For this review, take the finished solid that the model builds, in its own axes (mm). Face numbers are marked on the shaded views. Round coordinates to 2 decimals unless told otherwise and drop trailing zeros. Loops run counter-clockwise (first coordinate to the right, second up) from the corner with the lowest first, then second, coordinate; pieces in that order, holes last.
```python
from build123d import *

# Parameters (mm, degrees)
FILLET_4_R = 0.2
FILLET_5_R = 1


with BuildPart() as part:
    # Эскиз1 → Повернуть1 (revolve)
    with BuildSketch(Plane.XY, mode=Mode.PRIVATE) as revolve_1_sk:
        Polygon((-22.392450879, 1.834990157), (-22.392450879, 2.25), (-10.392450879, 2.25), (-9.392450879, 1.5), (-2.392450879, 1.5), (2.607549121, 1.05), (2.607549121, 0.75), (-2.663312046, 1.1), (-9.392450879, 1.1), (-10.602717789, 1.834990157), align=None)
    revolve(revolve_1_sk.sketch.rotate(Axis((-52.441675284, 0, 0), (1, 0, 0)), 90), axis=Axis((-52.441675284, 0, 0), (1, 0, 0)))

    # Скругление4
    fillet_4_edges = [part.edges().sort_by_distance(p)[0] for p in [
        (-22.392450879, 0, -2.25),
        (2.607549121, 0, -1.05),
    ]]
    fillet(fillet_4_edges, radius=FILLET_4_R)

    # Скругление5
    fillet_5_edges = [part.edges().sort_by_distance(p)[0] for p in [
        (-10.392450879, 0, -2.25),
        (-9.392450879, 0, -1.5),
    ]]
    fillet(fillet_5_edges, radius=FILLET_5_R)


solid = part.part
```
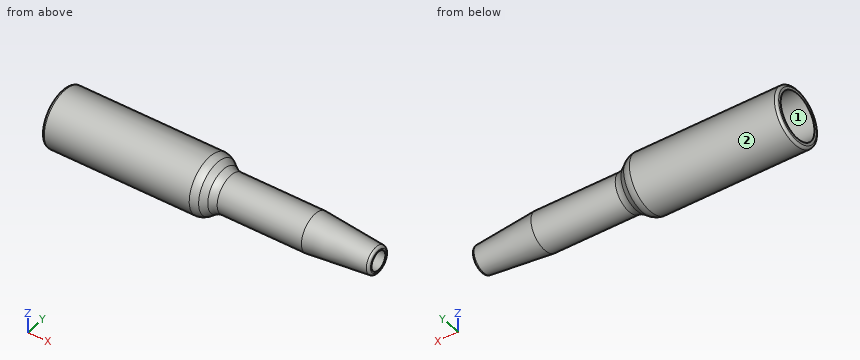
(1) Insertion check: pin 1 Ø1.5 at (x, z) = (-1.5, 1.5) entering from +Y. The pin has a flat end and moves straight along its axis. Give the tip position at first contact, or say it passes through.
(2) For L1, parallel to Y at x = -19.25, z = 0 (3 decimals); L2, parallel to Z at x = -20.5, y = -0.1; L3, parallel to Y at x = -7.5, z = 0, list the stretches that pass through material, from the lowest coordinate up.
(3) The part is to be moulded in two halves that separate along Z. For the marked faces 1 and 2, say which applies: pulls with the +Z half, pulls with the -Z half, needs draft (parallel to the pull), parting line crosses it, or undercut.
(4) Add section A-A (x = -1.25). Give the boundary of the cut face in (y, z), plus the area to 3 significant figures.
Outcome:
1. pin 1: stops at y = 1.21
2. L1: y = -2.25 to -1.835, 1.835 to 2.25
2. L2: z = -2.25 to -1.83, 1.83 to 2.25
2. L3: y = -1.5 to -1.1, 1.1 to 1.5
3. face 1: undercut
3. face 2: parting line crosses it
4. outline: circle Ø2.79 at (0, 0); hole circle Ø2.01 at (0, 0)
4. area: 2.95 mm2
